Autodesk Inventor part; units mm, degrees
ref_plane "YZ Plane" through (0, 0, 0) normal (1, 0, 0) x (0, 1, 0)
ref_plane "XZ Plane" through (0, 0, 0) normal (0, 1, 0) x (-1, 0, 0)
ref_plane "XY Plane" through (0, 0, 0) normal (0, 0, 1) x (1, 0, 0)
sketch "Sketch1" plane through (0, 0, 0) normal (0, 0, 1) x (1, 0, 0)
  circle A0 centre (0, 0) radius 0.5
  line L0 (-3, 72) -> (3, 72)
  line L1 (5, 70) -> (5, -1)
  line L2 (3, -3) -> (-3, -3)
  line L3 (-5, -1) -> (-5, 70)
  arc A1 (-3, 72) -> (-5, 70) centre (-3, 70) ccw
  arc A2 (5, 70) -> (3, 72) centre (3, 70) ccw
  arc A3 (-5, -1) -> (-3, -3) centre (-3, -1) ccw
  arc A4 (3, -3) -> (5, -1) centre (3, -1) ccw
  circle A5 centre (0, 67) radius 2.5
  line L4 (0, 72) -> (0, 61.8445)
  circle A6 centre (-3.25, 0) radius 0.5
  circle A7 centre (3.25, 0) radius 0.5
  point P0 (-5, 72)
  point P1 (-5, -3)
  point P2 (0, -3)
  dimension "d3" = 1
  dimension "d7" = 75
  dimension "d8" = 10
  dimension "d9" = 3
  dimension "d10" = 2
  dimension "d11" = 5
  dimension "d12" = 5
  dimension "d15" = 1
  dimension "d16" = 1
  dimension "d17" = 3.25
  dimension "d18" = 3.25
extrude "Extrusion1" add sketch "Sketch1" along normal blind 3
properties part number "FP V2 Servo Arm"
Design review of the part built by this model. Coordinates are the model's own, in mm. Coordinates: 2 decimals unless noted, no trailing zeros. Order: outer loops, then holes, each group sorted by start corner. A loop starts at its lowest first (then second) coordinate and runs counter-clockwise, first axis right, second up. Notation, with made-up numbers: (-6.5, 19.25) -> (50.5, 19.25) arc R23 ccw to (50.5, 27.25) -> close; hole circle Ø8 at (37.25, 76.5). An arc over 180 degrees is marked (long way). One line per item, written item: value. Start each with the question number.
Q1. Mouldability with a two-part tool opening along X and no side actions: class faces 1 (the cylindrical face through (1.15, 69.22, 1.48)), 2 (the flat face through (-5, 34, 1)), 3 (the flat face through (0, 35, 3)) as pulls with the +X half, pulls with the -X half, needs draft (parallel to the pull), parting line crosses it, or undercut.
Q2. Take a section at A-A, the plane z = 1.2. State the section outline as (x, y) points, then the cut area to 3 significant figures.
Q3. Insertion check: pin 1 Ø1.5 at (x, y) = (-3.5, 39) entering from -Z. The pin has a flat end and moves straight along its axis. Give the tip position at first contact, or say it passes through.
Q4. For probe 1 along Y at (x, z) = (3.25, 2); probe 2 along Y at (x, z) = (0, 1.6); probe 3 along Y at (x, z) = (1, 0.35), list the stretches that pass through material, from the lowest coordinate up.
Values follow:
1. face 1: undercut
1. face 2: pulls with the -X half
1. face 3: needs draft
2. outline: (-5, -1) arc R2 ccw to (-3, -3) -> (3, -3) arc R2 ccw to (5, -1) -> (5, 70) arc R2 ccw to (3, 72) -> (-3, 72) arc R2 ccw to (-5, 70) -> close; hole circle Ø1 at (-3.25, 0); hole circle Ø5 at (0, 67); hole circle Ø1 at (0, 0); hole circle Ø1 at (3.25, 0)
2. area: 725 mm2
3. pin 1: stops at z = 0
4. probe 1: y = -2.98 to -0.5, 0.5 to 71.98
4. probe 2: y = -3 to -0.5, 0.5 to 64.5, 69.5 to 72
4. probe 3: y = -3 to 64.71, 69.29 to 72
